Here's how the part is built. I have some questions about the finished solid (model axes, mm). A direction names the side the tool comes from. Coordinates: 2 decimals unless noted, no trailing zeros. Loops run counter-clockwise (first coordinate to the right, second up) from the corner with the lowest first, then second, coordinate; pieces in that order, holes last. Notation, with made-up numbers: (-29.75, 63) -> (21.25, 63) arc R17 ccw to (21.25, 84) -> close; hole circle Ø10 at (-10.75, 36.25). An arc over 180 degrees is marked (long way). Answer as a JSON object with one key per item and string values. Group by question number.
Q1. I want a section at D-D on x = 15. Count the separate pieces of the cut face and the enclosed holes in it, then the cut area to 3 significant figures.
Q2. I want a section at A-A on x = -21.7. Write out the boundary of the cut face in (y, z), then the cut area to 3 significant figures.
Q3. I want a section at C-C on y = 2.2. Write out the boundary of the cut face in (x, z), then the cut area to 3 significant figures.
Q4. On a 3-axis mill with a long thin cutter (end or side, diameter ignored), from which of +Z, -Z, +X, -X, +Y, -Y can I reach the whole of each face in a straight line? I mean faces 3 (the flat face through (0, 0, -26)), 4 (the flat face through (-28, 2, -16.5)). Say none if no direction works.
Q5. I'm going to push a flat-ended pin straight in: pin 1 (3 mm diameter, centred on x = -21.7, z = -30.5, fed in from -Y). Where does the tip first touch, or does it pass through?
Q6. Thinking about a two-plate mould opening in Z: for faces 1 (the flat face through (32.6, 2, 1)), 2 (the cylindrical face through (-20.52, 2.02, -31.79)), which applies, released by +Z, released by -Z, zero draft, split by the parting line, or undercut?
Q7. I want a section at B-B on z = -30.5. Write out the boundary of the cut face in (x, y).
Q8. I need wall thicknesses on line 1 (X direction, y = 2.3, z = 22); line 2 (Z direction, x = -5.5, y = 0.7); line 3 (Z direction, x = 14.5, y = 3.3). Which ranges of each line are inside material? Lowest first, please.
```python
from build123d import *

# Parameters (mm, degrees)
SKETCH1_W           = 65.2
SKETCH1_H           = 115
SKETCH1_R           = 1.75
SKETCH1_W_2         = 59
SKETCH1_H_2         = 64
BOSS_EXTRUDE1_DEPTH = 4
SKETCH2_R           = 1.75
CUT_EXTRUDE1_DEPTH  = 67.219408031
FILLET1_R           = 3
CHAMFER1_SIZE       = 0.4


with BuildPart() as part:
    # Sketch1 → Boss-Extrude1 (new body)
    with BuildSketch(Plane(origin=(0, 0, 0), x_dir=(1, 0, 0), z_dir=(0, 1, 0))):
        Rectangle(SKETCH1_W, SKETCH1_H)
        with Locations(Location((-15, 52.5, 0), (0, 0, 270))):
            Circle(SKETCH1_R, mode=Mode.SUBTRACT)
        with Locations(Location((15, 52.5, 0), (0, 0, 270))):
            Circle(SKETCH1_R, mode=Mode.SUBTRACT)
        with Locations(Location((15, -52.5, 0), (0, 0, 270))):
            Circle(SKETCH1_R, mode=Mode.SUBTRACT)
        with Locations(Location((-15, -52.5, 0), (0, 0, 270))):
            Circle(SKETCH1_R, mode=Mode.SUBTRACT)
        with Locations((0, -15.5)):
            Rectangle(SKETCH1_W_2, SKETCH1_H_2, mode=Mode.SUBTRACT)
    extrude(amount=BOSS_EXTRUDE1_DEPTH)

    # Sketch2 → Cut-Extrude1 (cut, through all)
    with BuildSketch(Plane(origin=(0, 4, 0), x_dir=(1, 0, 0), z_dir=(0, 1, 0))):
        with Locations((-21.7, 17.8)):
            Circle(SKETCH2_R)
        with Locations((21.7, 17.8)):
            Circle(SKETCH2_R)
        with Locations(Location((21.7, 30.5, 0), (0, 0, 270))):
            Circle(SKETCH2_R)
        with Locations(Location((-21.7, 30.5, 0), (0, 0, 270))):
            Circle(SKETCH2_R)
    extrude(amount=-CUT_EXTRUDE1_DEPTH, mode=Mode.SUBTRACT)

    # Fillet1
    fillet1_edges = [part.edges().sort_by_distance(p)[0] for p in [
        (20.528462549, 2, -16.5),
        (22.871537451, 2, -16.5),
        (-22.871537451, 2, -16.5),
        (-20.528462549, 2, -16.5),
    ]]
    fillet(fillet1_edges, radius=FILLET1_R)

    # Chamfer1
    chamfer1_edges = [part.edges().sort_by_distance(p)[0] for p in [
        (32.6, 4, 0),
        (-29.5, 0, 15.5),
        (0, 0, 47.5),
        (29.5, 0, 15.5),
        (27.817684603, 0, -16.5),
        (-29.5, 4, 15.5),
        (0, 4, -57.5),
        (0, 4, 47.5),
        (29.5, 4, 15.5),
        (27.817684603, 4, -16.5),
        (-15, 0, -54.25),
        (-15, 4, -54.25),
        (15, 0, -54.25),
        (15, 4, -54.25),
        (15, 0, 50.75),
        (15, 4, 50.75),
        (-15, 0, 50.75),
        (-15, 4, 50.75),
        (-32.6, 4, 0),
        (0, 0, -57.5),
        (32.6, 0, 0),
        (0, 0, 57.5),
        (-32.6, 0, 0),
        (-21.7, 0, -32.25),
        (-21.7, 4, -32.25),
        (21.7, 0, -32.25),
        (21.7, 4, -32.25),
        (21.7, 4, -19.55),
        (21.7, 0, -19.55),
        (-21.7, 4, -19.55),
        (0, 4, -16.5),
        (-27.817684603, 4, -16.5),
        (-24.435524013, 4, -17.028052121),
        (-18.964475987, 4, -17.028052121),
        (18.964475987, 4, -17.028052121),
        (24.435524013, 4, -17.028052121),
        (0, 0, -16.5),
        (-21.7, 0, -19.55),
        (-27.817684603, 0, -16.5),
        (-24.435524013, 0, -17.028052121),
        (-18.964475987, 0, -17.028052121),
        (18.964475987, 0, -17.028052121),
        (24.435524013, 0, -17.028052121),
        (0, 4, 57.5),
    ]]
    chamfer(chamfer1_edges, length=CHAMFER1_SIZE)


solid = part.part
```
Result set:
{
 "1": {"separate pieces": "4", "enclosed holes": "0", "area": "175 mm²"},
 "2": {"outline": "(0, -57.1) -> (0.4, -57.5) -> (3.6, -57.5) -> (4, -57.1) -> (4, -32.65) -> (3.6, -32.25) -> (0.4, -32.25) -> (0, -32.65) -> close; (0, -28.35) -> (0.4, -28.75) -> (3.6, -28.75) -> (4, -28.35) -> (4, -19.95) -> (3.6, -19.55) -> (0.4, -19.55) -> (0, -19.95) -> close; (0, 47.9) -> (0.4, 47.5) -> (3.6, 47.5) -> (4, 47.9) -> (4, 57.1) -> (3.6, 57.5) -> (0.4, 57.5) -> (0, 57.1) -> close", "area": "177 mm²"},
 "3": {"outline": "(-32.6, -57.5) -> (32.6, -57.5) -> (32.6, 57.5) -> (-32.6, 57.5) -> close; hole (-29.5, -16.5) -> (-26.14, -16.5) arc R3 cw to (-23.33, -18.43) arc R1.75 ccw to (-20.07, -18.43) arc R3 cw to (-17.26, -16.5) -> (17.26, -16.5) arc R3 cw to (20.07, -18.43) arc R1.75 ccw to (23.33, -18.43) arc R3 cw to (26.14, -16.5) -> (29.5, -16.5) -> (29.5, 47.5) -> (-29.5, 47.5) -> close; hole circle Ø3.5 at (-21.7, -30.5); hole circle Ø3.5 at (-15, -52.5); hole circle Ø3.5 at (-15, 52.5); hole circle Ø3.5 at (15, -52.5); hole circle Ø3.5 at (15, 52.5); hole circle Ø3.5 at (21.7, -30.5)", "area": "3,640 mm²"},
 "4": {"face 3": "+Z, -Z, +X, -X, -Y", "face 4": "+Y, -Y"},
 "5": {"pin 1": "passes through"},
 "6": {"face 1": "zero draft", "face 2": "undercut"},
 "7": {"outline": "(-32.6, 0.4) -> (-32.2, 0) -> (-23.85, 0) -> (-23.45, 0.4) -> (-23.45, 3.6) -> (-23.85, 4) -> (-32.2, 4) -> (-32.6, 3.6) -> close; (-19.95, 0.4) -> (-19.55, 0) -> (19.55, 0) -> (19.95, 0.4) -> (19.95, 3.6) -> (19.55, 4) -> (-19.55, 4) -> (-19.95, 3.6) -> close; (23.45, 0.4) -> (23.85, 0) -> (32.2, 0) -> (32.6, 0.4) -> (32.6, 3.6) -> (32.2, 4) -> (23.85, 4) -> (23.45, 3.6) -> close"},
 "8": {"line 1": "x = -32.6 to -29.5, 29.5 to 32.6", "line 2": "z = -57.5 to -16.5, 47.5 to 57.5", "line 3": "z = -57.5 to -54.18, -50.82 to -16.5, 47.5 to 50.82, 54.18 to 57.5"}
}
